from build123d import *

# Parameters (mm, degrees)
ESQUISSE1_W                 = 22
ESQUISSE1_H                 = 25
BOSS_EXTRU_1_DEPTH          = 45
BOSS_EXTRU_2_DEPTH          = 5
BOSS_EXTRU_3_DEPTH          = 50
D_GAGEMENT_1_41_D           = 6.7564
D_GAGEMENT_1_41_CSINK_D     = 8.0264
D_GAGEMENT_1_41_CSINK_ANGLE = 90
CONG_1_SIZE                 = 3


with BuildPart() as part:
    # Esquisse1 → Boss.-Extru.1 (new body)
    with BuildSketch(Plane.XY):
        with Locations((-77.82148747, 16.657061647)):
            Rectangle(ESQUISSE1_W, ESQUISSE1_H)
    extrude(amount=BOSS_EXTRU_1_DEPTH)

    # Esquisse2 → Boss.-Extru.2 (add)
    with BuildSketch(Plane(origin=(0, 29.157061647, 0), x_dir=(1, 0, 0), z_dir=(0, 1, 0))):
        Polygon((-85.32148747, -18.169872981), (-85.32148747, -26.830127019), (-77.82148747, -31.160254038), (-70.32148747, -26.830127019), (-70.32148747, -18.169872981), (-77.82148747, -13.839745962), align=None)
    extrude(amount=BOSS_EXTRU_2_DEPTH)

    # Esquisse4 → Boss.-Extru.3 (add)
    # profile 1 of 2: a face of its own
    with BuildSketch(Plane(origin=(0, 34.157061647, 0), x_dir=(1, 0, 0), z_dir=(0, 1, 0))):
        Polygon((-71.82148747, -12), (-63.82148747, -20), (-63.82148747, -47), (-91.82148747, -47), (-91.82148747, -20), (-83.82148747, -12), align=None)
        Polygon((-77.82148747, -13.839745962), (-85.32148747, -18.169872981), (-85.32148747, -26.830127019), (-77.82148747, -31.160254038), (-70.32148747, -26.830127019), (-70.32148747, -18.169872981), align=None, mode=Mode.SUBTRACT)
    # profile 2 of 2: a face of its own
    with BuildSketch(Plane(origin=(0, 34.157061647, 0), x_dir=(1, 0, 0), z_dir=(0, 1, 0))):
        Polygon((-70.32148747, -18.169872981), (-77.82148747, -13.839745962), (-85.32148747, -18.169872981), (-85.32148747, -26.830127019), (-77.82148747, -31.160254038), (-70.32148747, -26.830127019), align=None)
    extrude(amount=BOSS_EXTRU_3_DEPTH)

    # Dégagement 1/41 (through all)
    with Locations(Plane(origin=(0, 0, 0), x_dir=(-1, 0, 0), z_dir=(0, 0, -1))):
        with Locations((77.82148747, 16.657061647)):
            CounterSinkHole(D_GAGEMENT_1_41_D / 2, D_GAGEMENT_1_41_CSINK_D / 2, counter_sink_angle=D_GAGEMENT_1_41_CSINK_ANGLE)

    # Congé1
    # a fillet whose section is not a circle: 3 mm, written as the material it takes off along each edge
    with BuildSketch(Plane(origin=(-88.82148747, 4.157061647, -7.5), x_dir=(1, 0, 0), z_dir=(0, 0, 1)), Plane(origin=(-66.82148747, 29.157061647, -7.5), x_dir=(-1, 0, 0), z_dir=(0, 0, 1)), Plane(origin=(-66.82148747, 4.157061647, -7.5), x_dir=(0, 1, 0), z_dir=(0, 0, 1))) as cong_1_piece_1:
        with BuildLine():
            Bezier((CONG_1_SIZE, 0), (0, 0), (0, CONG_1_SIZE), weights=[1, 0.212132034, 1])
            Line((0, CONG_1_SIZE), (0, 0))
            Line((0, 0), (CONG_1_SIZE, 0))
        make_face()
    extrude(amount=60, mode=Mode.SUBTRACT)
    with BuildSketch(Plane(origin=(-88.82148747, 29.157061647, -7.5), x_dir=(1, 0, 0), z_dir=(0, 0, 1))) as cong_1_piece_2:
        with BuildLine():
            Bezier((CONG_1_SIZE, 0), (0, 0), (0, -CONG_1_SIZE), weights=[1, 0.212132034, 1])
            Line((0, -CONG_1_SIZE), (0, 0))
            Line((0, 0), (CONG_1_SIZE, 0))
        make_face()
    extrude(amount=60, mode=Mode.SUBTRACT)


solid = part.part
Part model, mm, in its own coordinate system. A direction names the side the tool comes from. Give positions to 0.01 mm unless a question says otherwise; leave off trailing zeros. Loops run counter-clockwise (first coordinate to the right, second up) from the corner with the lowest first, then second, coordinate; pieces in that order, holes last.
(1) Pin check, flat tips, straight feed: pin 1 (6 mm diameter, centred on x = -78, y = 60, fed in from -Z); pin 2 (15 mm diameter, centred on y = 15, z = 30.5, fed in from +X); pin 3 (1.5 mm diameter, centred on y = 32, z = 22, fed in from +X). Stop position of each tip, or through.
Return value:
pin 1: stops at z = 12
pin 2: stops at x = -66.82
pin 3: stops at x = -70.32
(2) Band-saw the part on A-A (y = 46). Write the cut outline in (x, z), and give its area (3 significant figures).
Return value:
outline: (-91.82, 20) - (-83.82, 12) - (-71.82, 12) - (-63.82, 20) - (-63.82, 47) - (-91.82, 47) - close
area: 916 mm2
(3) Pull direction X, two halves, no side cores. Call faces 5 (the flat face through (-78, 59, 12)), 6 (the cylindrical face through (-81.196, 16.806, 23.128)), 7 (the flat face through (-87.88, 58.81, 16.06)): pulls with the +X half, pulls with the -X half, needs draft (parallel to the pull), parting line crosses it, or undercut.
Return value:
face 5: needs draft
face 6: undercut
face 7: pulls with the -X half
(4) Band-saw the part on D-D (y = 9.5). Write the cut outline in (x, z), and give its area (3 significant figures).
Return value:
outline: (-88.82, 0) - (-66.82, 0) - (-66.82, 45) - (-88.82, 45) - close
area: 990 mm2
(5) Drill centre lines: line 1 along X through (y, z) = (16.5, 18); line 2 along Y through (x, z) = (-80.75, 37.5); line 3 along Y through (x, z) = (-73.5, 30). Where is each one in solid material? Low to high.
Return value:
line 1: x = -88.82 to -81.2, -74.45 to -66.82
line 2: y = 4.16 to 14.97, 18.34 to 29.16, 34.16 to 84.16
line 3: y = 4.16 to 29.16, 34.16 to 84.16
(6) Band-saw the part on C-C (y = 32.5). Write the cut outline in (x, z).
Return value:
outline: (-85.32, 18.17) - (-77.82, 13.84) - (-70.32, 18.17) - (-70.32, 26.83) - (-77.82, 31.16) - (-85.32, 26.83) - close
(7) 3-axis set-ups, long thin cutter, end or side, ignore diameter. For faces 1 (the flat face through (-85.321, 32, 22)), 2 (the flat face through (-66.821, 17, 22)), 3 (the flat face through (-70.321, 32, 23)), 4 (the flat face through (-74.124, 31.622, 29.026)): which of +Z, -Z, +X, -X, +Y, -Y reach the whole face in a straight line?
Return value:
face 1: +Z, -Z, -X
face 2: +Z, -Z, +X, -Y
face 3: +Z, -Z, +X
face 4: +Z, +X
(8) Band-saw the part on B-B (z = 41). Count the separate pieces of the cut face and the enclosed holes in it, and give its area (3 significant figures).
Return value:
separate pieces: 2
enclosed holes: 1
area: 1,900 mm2
